from build123d import *

# Parameters (mm, degrees)
SKETCH1_R                = 35
SKETCH1_R_2              = 30
BOSS_EXTRUDE1_DEPTH      = 30
BOSS_EXTRUDE2_DEPTH      = 6
M5_CLEARANCE_HOLE1_D     = 5.5
M5_CLEARANCE_HOLE1_DEPTH = 10
M5_CLEARANCE_HOLE1_TIP   = 1.652366702


with BuildPart() as part:
    # Sketch1 → Boss-Extrude1 (new body)
    with BuildSketch(Plane(origin=(0, 0, 0), x_dir=(1, 0, 0), z_dir=(0, 1, 0))):
        with Locations(Location((0, 0, 0), (0, 0, 270))):
            Circle(SKETCH1_R)
        with Locations(Location((0, 0, 0), (0, 0, 270))):
            Circle(SKETCH1_R_2, mode=Mode.SUBTRACT)
    extrude(amount=BOSS_EXTRUDE1_DEPTH)

    # Sketch2 → Boss-Extrude2 (add)
    with BuildSketch(Plane.XZ):
        with BuildLine():
            Line((0, -35), (-45, -35))
            Line((-45, -35), (-45, 35))
            Line((-45, 35), (0, 35))
            ThreePointArc((0, 35), (-35, 0), (0, -35))
        make_face()
    extrude(amount=-BOSS_EXTRUDE2_DEPTH)

    # M5 Clearance Hole1
    with Locations(Plane(origin=(0, 6, 0), x_dir=(1, 0, 0), z_dir=(0, 1, 0))):
        with Locations((-35, 25), (-35, -25)):
            Hole(M5_CLEARANCE_HOLE1_D / 2, depth=M5_CLEARANCE_HOLE1_DEPTH)
            with Locations((0, 0, -(M5_CLEARANCE_HOLE1_DEPTH + M5_CLEARANCE_HOLE1_TIP / 2))):  # 118° drill point
                Cone(0, M5_CLEARANCE_HOLE1_D / 2, M5_CLEARANCE_HOLE1_TIP, mode=Mode.SUBTRACT)


solid = part.part
For this review, take the finished solid that the model builds, in its own axes (mm). A direction names the side the tool comes from. Round coordinates to 2 decimals unless told otherwise and drop trailing zeros. Order: outer loops, then holes, each group sorted by start corner. A loop starts at its lowest first (then second) coordinate and runs counter-clockwise, first axis right, second up. Notation, with made-up numbers: (-1.75, 12) -> (28.25, 12) arc R25 ccw to (28.25, 31) -> close; hole circle Ø2 at (-33.5, 21.25). An arc over 180 degrees is marked (long way). Write item = value, one per line. Start each with the question number.
1) Tool access review of faces 1 (the face through (-37, 6, 0)), 2 (the face through (-32.253, 2.958, -25.121)), 3 (the face through (34.7, 14.79, -4.56)): name each direction out of +Z, -Z, +X, -X, +Y, -Y from which nothing blocks a thin tool from reaching the whole face with its end or side.
2) Take a section at D-D on z = 17. State the section outline as (x, y) points.
3) Take a section at B-B on x = 21. State the section outline as (y, z) points.
4) Take a section at C-C on y = 10. State the section outline as (x, z) points.
5) To check wall thickness, follow line 1 (Z direction, x = -35, y = 1.75); line 2 (X direction, y = 3.15, z = -25); line 3 (X direction, y = 4, z = 22.5). State the ranges of each line that lie inside material, in increasing order. Write a range as from..to.
6) Insertion check: pin 1 (10 mm diameter, centred on x = 6, y = 12.5, fed in from +Z); pin 2 (4 mm diameter, centred on y = 7, z = -2.5, fed in from +X); pin 3 (4 mm diameter, centred on x = 6.5, y = 16, fed in from +Z). Each pin has a flat end and moves straight along its axis. Give the tip position at first contact, or say it passes through.
7) Take a section at A-A on z = -25. State the section outline as (x, y) points, plus the area to 3 significant figures.
Verdict:
q1.face_1 = -X, +Y
q1.face_2 = +Y, -Y
q1.face_3 = +Y
q2.outline = (-45, 0) -> (-24.72, 0) -> (-24.72, 30) -> (-30.59, 30) -> (-30.59, 6) -> (-45, 6) -> close; (24.72, 0) -> (30.59, 0) -> (30.59, 30) -> (24.72, 30) -> close
q3.outline = (0, -28) -> (30, -28) -> (30, -21.42) -> (0, -21.42) -> close; (0, 21.42) -> (30, 21.42) -> (30, 28) -> (0, 28) -> close
q4.outline = circle Ø70 at (0, 0); hole circle Ø60 at (0, 0)
q5.line_1 = -35..-27.75, -22.25..22.25, 27.75..35
q5.line_2 = -45..-37.75, -32.25..-16.58, 16.58..24.49
q5.line_3 = -45..-36.15, -33.85..-19.84, 19.84..26.81
q6.pin_1 = 34.99
q6.pin_2 = 35
q6.pin_3 = 34.71
q7.outline = (-45, 0) -> (-37.75, 0) -> (-37.75, 6) -> (-45, 6) -> close; (-32.25, 0) -> (-16.58, 0) -> (-16.58, 30) -> (-24.49, 30) -> (-24.49, 6) -> (-32.25, 6) -> close; (16.58, 0) -> (24.49, 0) -> (24.49, 30) -> (16.58, 30) -> close
q7.area = 565 mm2
